Verification items for the finished model (mm, model axes). A direction names the side the tool comes from. Give positions to 0.01 mm unless a question says otherwise; leave off trailing zeros. Write each loop counter-clockwise with the first axis right and the second up, starting at its lowest first coordinate (ties: lowest second). Pieces come first, ordered by that corner, then holes. Notation, with made-up numbers: (15, 57) - (40, 57) arc R15 cw to (40, 69) - close; hole circle Ø11 at (-23.75, 64.25). An arc over 180 degrees is marked (long way). Answer as a JSON object with one key per item and string values. Group by question number.
Item 1: Sectioned sample at C-C, the plane y = -3. Record the boundary of the cut face in (x, z), and give its area (3 significant figures).
Item 2: Sectioned sample at A-A, the plane z = 0. Record the boundary of the cut face in (x, y).
Item 3: Scan lines: line 1 along X through (y, z) = (-1, 0.25); line 2 along Z through (x, y) = (-21, -6); line 3 along Z through (x, y) = (0, -3). Record each from-to range of solid material in increasing order. Write a range as [from, to].
Item 4: Tool access check on faces 4 (the face through (32.5, -3, 0)), 5 (the face through (23, -4, 2.158)). Record the directions out of +Z, -Z, +X, -X, +Y, -Y that give a thin tool (end or side, any length) a straight path to the whole face; none if there is none.
Item 5: Sectioned sample at B-B, the plane x = 0. Record the boundary of the cut face in (y, z), and give its area (3 significant figures).
Item 6: Draft check along Z on faces 1 (the face through (0, -3, -12)), 2 (the face through (-30.789, -3.549, 10.196)), 3 (the face through (5.97, -3.45, 9.36)). Enter one of: +Z half, -Z half, draft (parallel to the pull), parting line (faces both ways), or undercut.
Item 7: Sectioned sample at D-D, the plane x = -22. Record the boundary of the cut face in (y, z).
```python
from build123d import *

# Parameters (mm, degrees)
F0_W     = 65
F0_H     = 24
F0_R     = 11.1
F1_DEPTH = 7
F2_R     = 6
F3_W     = 11.910181
F3_H     = 4.31511
F4_DEPTH = 7.001


with BuildPart() as f1:
    # F0 (on Front) → F1 (new body)
    with BuildSketch(Plane.XZ):
        Rectangle(F0_W, F0_H)
        Circle(F0_R, mode=Mode.SUBTRACT)
    extrude(amount=F1_DEPTH)

    # F2
    f2_edges = [f1.edges().sort_by_distance(p)[0] for p in [
        (-32.5, -3.5, 12),
        (-32.5, -3.5, -12),
        (32.5, -3.5, -12),
        (32.5, -3.5, 12),
    ]]
    fillet(f2_edges, radius=F2_R)

    # F3 (on face) → F4 (cut, through all)
    with BuildSketch(Plane.XZ.offset(7)):
        with Locations((-23.196599, 0)):
            Rectangle(F3_W, F3_H)
        with Locations((23.196599, 0)):
            Rectangle(F3_W, F3_H)
    extrude(amount=-F4_DEPTH, mode=Mode.SUBTRACT)


solid = f1.part
```
Geometry check:
{
 "1": {"outline": "(-32.5, -6) arc R6 ccw to (-26.5, -12) - (26.5, -12) arc R6 ccw to (32.5, -6) - (32.5, 6) arc R6 ccw to (26.5, 12) - (-26.5, 12) arc R6 ccw to (-32.5, 6) - close; hole (-29.15, -2.16) - (-17.24, -2.16) - (-17.24, 2.16) - (-29.15, 2.16) - close; hole circle Ø22.2 at (0, 0); hole (17.24, -2.16) - (29.15, -2.16) - (29.15, 2.16) - (17.24, 2.16) - close", "area": "1,040 mm^2"},
 "2": {"outline": "(-32.5, -7) - (-29.15, -7) - (-29.15, 0) - (-32.5, 0) - close; (-17.24, -7) - (-11.1, -7) - (-11.1, 0) - (-17.24, 0) - close; (11.1, -7) - (17.24, -7) - (17.24, 0) - (11.1, 0) - close; (29.15, -7) - (32.5, -7) - (32.5, 0) - (29.15, 0) - close"},
 "3": {"line 1": "[-32.5, -29.15], [-17.24, -11.1], [11.1, 17.24], [29.15, 32.5]", "line 2": "[-12, -2.16], [2.16, 12]", "line 3": "[-12, -11.1], [11.1, 12]"},
 "4": {"face 4": "+Z, -Z, +X, +Y, -Y", "face 5": "+Y, -Y"},
 "5": {"outline": "(-7, -12) - (0, -12) - (0, -11.1) - (-7, -11.1) - close; (-7, 11.1) - (0, 11.1) - (0, 12) - (-7, 12) - close", "area": "12.6 mm^2"},
 "6": {"face 1": "-Z half", "face 2": "+Z half", "face 3": "undercut"},
 "7": {"outline": "(-7, -12) - (0, -12) - (0, -2.16) - (-7, -2.16) - close; (-7, 2.16) - (0, 2.16) - (0, 12) - (-7, 12) - close"}
}
